Work out the finished part from the listing and answer in its coordinate system (mm). A direction names the side the tool comes from. Round coordinates to 2 decimals unless told otherwise and drop trailing zeros. Order: outer loops, then holes, each group sorted by start corner. A loop starts at its lowest first (then second) coordinate and runs counter-clockwise, first axis right, second up. Notation, with made-up numbers: (33.5, 31.25) - (73.5, 31.25) arc R25 ccw to (73.5, 59.25) - close; hole circle Ø3 at (36, 25). An arc over 180 degrees is marked (long way). Use one line per item in the form item = value. Start each with the question number.
Q1. For a pull along Z with two mould halves and no side action, classify faces 1 (the flat face through (0, -8, -2.05)), 2 (the cylindrical face through (3.648, -6.361, 1.113)), 3 (the flat face through (-3.2, -5.4, 2)) as +Z half, -Z half, draft (parallel to the pull), parting line (faces both ways), or undercut.
Q2. The part is cut by section A-A on x = 0. Determine the outline of the cut face in (y, z), plus the area to 3 significant figures.
Q3. Find the intervals of material crossed by line 1 (Y direction, x = 0, z = -3.3); line 2 (X direction, y = -7.23, z = 0.8); line 3 (Z direction, x = -11, y = -3.5), in increasing order. Write a range as [from, to].
Q4. The part is cut by section D-D on x = -3.25. Determine the outline of the cut face in (y, z).
Q5. Which of the six approach directions +Z, -Z, +X, -X, +Y, -Y give full straight-line access (tool end or side, diameter ignored) to faces 4 (the flat face through (-7.734, -7.095, -0.835)), 5 (the cylindrical face through (-4.488, -6.899, -0.916)), 6 (the flat face through (-7.269, -2.514, -0.835))?
Q6. Given P1, Ø1, axis at y = -1.5, z = 0, coming from the -X side; P2, Ø2, axis at x = -5.5, z = 0.5, coming from the +Y side; P3, Ø6, axis at x = 0, y = -7, coming from the +Z side, each flat-ended and moving along its own axis, determine where each tip first touches the part or whether it passes through.
Q7. The part is cut by section B-B on z = -1.5. Determine the outline of the cut face in (x, y).
Q8. The part is cut by section C-C on y = -7.23. Determine the outline of the cut face in (x, z).
Autodesk Inventor part; units mm, degrees
ref_plane "YZ Plane" through (0, 0, 0) normal (1, 0, 0) x (0, 1, 0)
ref_plane "XZ Plane" through (0, 0, 0) normal (0, 1, 0) x (-1, 0, 0)
ref_plane "XY Plane" through (0, 0, 0) normal (0, 0, 1) x (1, 0, 0)
sketch "Sketch1" plane through (0, 0, 0) normal (0, 0, 1) x (1, 0, 0)
  circle A0 centre (0, -7.23) radius 0.5
  circle A1 centre (0, -7.23) radius 3.75
  point P0 (0, 0)
  dimension "d0" = 7.5
extrude "Extrusion1" add sketch "Sketch1" along normal blind 2
ref_plane "Work Plane1" through (0, 0, -1.75) normal (0, 0, -1) x (-1, 0, 0)
sketch "Sketch2" plane through (0, 0, -1.75) normal (0, 0, -1) x (-1, 0, 0)
  circle A0 centre (0, -7.23) radius 0.5
  circle A1 centre (0, -7.23) radius 3.75
  circle A2 centre (0, -7.23) radius 0.5
  point P0 (0, 0)
extrude "Extrusion2" add sketch "Sketch2" along normal blind 2
sketch "Sketch3" plane through (0, -7.23, 2) normal (0, 0, 1) x (1, 0, 0)
  line L0 (-1.7434, -1.6216) -> (-2.9, 11.6822) construction
  arc A0 (-1.7434, -1.6216) -> (1.7434, -1.6216) centre (0, -1.47) ccw construction
  line L1 (1.7434, -1.6216) -> (2.9, 11.6822) construction
  arc A1 (2.9, 11.6822) -> (-2.9, 11.6822) centre (0, 13.98) ccw construction
  circle A2 centre (0, 13.98) radius 2.7 construction
  circle A3 centre (0, 6.21) radius 0.5 construction
  circle A4 centre (0, 8.28) radius 0.5 construction
  circle A5 centre (0, -2.07) radius 0.5 construction
  circle A6 centre (0, 0) radius 0.5 construction
  circle A7 centre (0, 2.07) radius 0.5 construction
  circle A8 centre (0, 4.14) radius 0.5 construction
  circle A9 centre (0, 0) radius 3.75
  circle A10 centre (0, 0) radius 3.75
  line L2 (-2.9991, 2.2512) -> (-11.6594, 7.2512)
  line L3 (-1.875, -3.2476) -> (-13.7594, 3.6139)
  line L4 (-12.9585, 11.9353) -> (6.9601, 0.4353)
  line L5 (-11.6594, 7.2512) -> (-13.7594, 3.6139)
  point P0 (0, 7.23)
  point P1 (-1.875, -3.2476)
  dimension "d5" = 90
  dimension "d6" = 4.2
  dimension "d7" = 10
extrude "Extrusion3" add sketch "Sketch3" against normal up to surface (5.75 mm away) contours A9 L3 L5 L2
sketch "Sketch4" plane through (-11.6594, 0.0212, 2) normal (0.5, 0.866, 0) x (0.866, -0.5, 0)
  line L0 (10, 5.75) -> (0, 5.75)
  line L1 (0, 0) -> (0, 5.75)
  line L2 (10, 0) -> (0, 0)
  line L3 (10, 2) -> (10, 0)
  line L4 (10, 2) -> (10, 3.75)
  line L5 (10, 5.75) -> (10, 3.75)
  circle A0 centre (2.5, 3) radius 1.6
  point P0 (10.1079, 2)
  dimension "d10" = 3.2
  dimension "d11" = 2.5
  dimension "d12" = 3
extrude "Extrusion4" cut sketch "Sketch4" against normal through all contours A0
sketch "Sketch5" plane through (0, 0, -1.75) normal (0, 0, 1) x (1, 0, 0)
  arc A0 (-1.875, -10.4776) -> (-2.9991, -4.9788) centre (0, -7.23) ccw construction
  circle A1 centre (0, -7.23) radius 0.5 construction
  circle A2 centre (0, -7.23) radius 4.5
  point P0 (0, 0)
  dimension "d15" = 9
extrude "Extrusion5" cut sketch "Sketch5" along normal blind 2 and the other way blind 0.3
properties part number "Palanca servo_dedo_1"
Found:
q1.face_1 = undercut
q1.face_2 = draft
q1.face_3 = +Z half
q2.outline = (-10.98, -3.75) - (-7.73, -3.75) - (-7.73, -2.05) - (-10.98, -2.05) - close; (-10.98, 0.25) - (-7.73, 0.25) - (-7.73, 2) - (-10.98, 2) - close; (-6.73, -3.75) - (-3.48, -3.75) - (-3.48, -2.05) - (-6.73, -2.05) - close; (-6.73, 0.25) - (-3.48, 0.25) - (-3.48, 2) - (-6.73, 2) - close
q2.area = 22.4 mm²
q3.line_1 = [-10.98, -7.73], [-6.73, -3.48]
q3.line_2 = [-7.5, -0.5], [0.5, 3.75]
q3.line_3 = [-3.75, -2.59], [0.59, 2]
q4.outline = (-9.68, -3.75) - (-4.83, -3.75) - (-4.83, -2.05) - (-9.68, -2.05) - close; (-9.68, 0.25) - (-4.83, 0.25) - (-4.83, 2) - (-9.68, 2) - close
q5.face_4 = +Z, -Z, -X, -Y
q5.face_5 = +X
q5.face_6 = +Z, -Z, +Y
q6.P1 = -12.83
q6.P2 = -2.96
q6.P3 = 2
q7.outline = (-13.76, -3.62) - (-12.91, -4.11) - (-10.81, -0.47) - (-11.66, 0.02) - close; (-10.28, -5.63) - (-4.03, -9.23) arc R4.5 cw to (-3.65, -4.6) - (-8.18, -1.99) - close
q8.outline = (-7.5, -3.75) - (-0.5, -3.75) - (-0.5, -2.05) - (-4.5, -2.05) - (-4.5, 0.25) - (-0.5, 0.25) - (-0.5, 2) - (-7.5, 2) - close; (0.5, -3.75) - (3.75, -3.75) - (3.75, -2.05) - (0.5, -2.05) - close; (0.5, 0.25) - (3.75, 0.25) - (3.75, 2) - (0.5, 2) - close
